For this review, take the finished solid that the model builds, in its own axes (mm). Face numbers are marked on the shaded views. A direction names the side the tool comes from. Coordinates: 2 decimals unless noted, no trailing zeros. Write each loop counter-clockwise with the first axis right and the second up, starting at its lowest first coordinate (ties: lowest second). Pieces come first, ordered by that corner, then holes. Notation, with made-up numbers: (4.25, -33.75) - (32.25, -33.75) arc R23 ccw to (32.25, -12.75) - close; hole circle Ø8 at (-18.75, 22.5). An arc over 180 degrees is marked (long way). Use one line per item in the form item = value. Start each with the question number.
1) We need section A-A (z = 31). Give the boundary of the cut face in (x, y), plus the area to 3 significant figures.
2) We need section D-D (x = 18.5). Give the boundary of the cut face in (y, z).
3) We need section C-C (y = -50). Give the boundary of the cut face in (x, z).
4) We need section B-B (x = 28.5). Give the boundary of the cut face in (y, z), plus the area to 3 significant figures.
5) For L1, parallel to X at y = -42, z = 25.5; L2, parallel to Z at x = 41.5, y = -10; L3, parallel to Y at x = 12, z = 3, list the stretches that pass through material, from the lowest coordinate up. Write a range as from..to.
6) Insertion check: P1, Ø3, axis at x = 32, y = -17, coming from the -Z side; P2, Ø19, axis at x = 39, z = 34, coming from the -Y side; P3, Ø5.5, axis at y = -21, z = 30.5, coming from the -X side; P4, Ø5, axis at x = 30.5, y = -36, coming from the +Z side. Each pin has a flat end and moves straight along its axis. Give the tip position at first contact, or say it passes through.
7) Tool access review of the marked faces 4, 5, 6 and 7: name each direction out of +Z, -Z, +X, -X, +Y, -Y from which nothing blocks a thin tool from reaching the whole face with its end or side.
8) Mouldability with a two-part tool opening along Y and no side actions: class the marked faces 1, 2 and 3 as pulls with the +Y half, pulls with the -Y half, needs draft (parallel to the pull), parting line crosses it, or undercut.
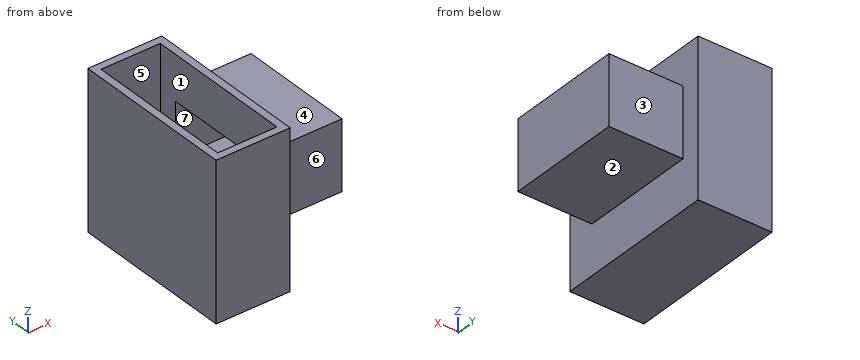
```python
from build123d import *

# Parameters (mm, degrees)
F0_W     = 35.9010435641
F0_H     = 59.8467253149
F1_DEPTH = 25.4
F2_W     = 56.2424324453
F2_H     = 53.3904395998
F3_DEPTH = 25.4
F4_W     = 39.9578805082
F4_H     = 23.749506101
F5_DEPTH = 25.4
F6_T     = -2.54


with BuildPart() as f1:
    # F0 (on Top) → F1 (new body)
    with BuildSketch(Plane.XY):
        with Locations((-17.950521782, 29.9233626574)):
            Rectangle(F0_W, F0_H)
    extrude(amount=F1_DEPTH)


with BuildPart() as f3:
    # F2 (on Right) → F3 (new body)
    with BuildSketch(Plane.YZ):
        with Locations((-28.1212162226, 26.6952197999)):
            Rectangle(F2_W, F2_H)
    extrude(amount=F3_DEPTH)

    # F4 (on face) → F5 (join)
    with BuildSketch(Plane.YZ.offset(25.4)):
        with Locations((-26.5757592861, 28.7435064092)):
            Rectangle(F4_W, F4_H)
    extrude(amount=F5_DEPTH)

    # F6
    f6_openings = [f3.faces().sort_by_distance(p)[0] for p in [
        (12.7, -28.121216, 53.39044),
    ]]
    offset(amount=F6_T, openings=f6_openings, kind=Kind.INTERSECTION)


solid = f3.part
```
Determined:
q1.outline = (0, -56.24) - (25.4, -56.24) - (25.4, -46.55) - (50.8, -46.55) - (50.8, -6.6) - (25.4, -6.6) - (25.4, 0) - (0, 0) - close; hole (2.54, -53.7) - (22.86, -53.7) - (22.86, -44.01) - (48.26, -44.01) - (48.26, -9.14) - (22.86, -9.14) - (22.86, -2.54) - (2.54, -2.54) - close
q1.area = 518 mm²
q2.outline = (-56.24, 0) - (0, 0) - (0, 53.39) - (-2.54, 53.39) - (-2.54, 2.54) - (-53.7, 2.54) - (-53.7, 53.39) - (-56.24, 53.39) - close
q3.outline = (0, 0) - (25.4, 0) - (25.4, 53.39) - (22.86, 53.39) - (22.86, 2.54) - (2.54, 2.54) - (2.54, 53.39) - (0, 53.39) - close
q4.outline = (-46.55, 16.87) - (-6.6, 16.87) - (-6.6, 40.62) - (-46.55, 40.62) - close; hole (-44.01, 19.41) - (-9.14, 19.41) - (-9.14, 38.08) - (-44.01, 38.08) - close
q4.area = 298 mm²
q5.L1 = 0..2.54, 48.26..50.8
q5.L2 = 16.87..19.41, 38.08..40.62
q5.L3 = -56.24..-53.7, -2.54..0
q6.P1 = 16.87
q6.P2 = -46.55
q6.P3 = 0
q6.P4 = 40.62
q7.face_4 = +Z, +X, +Y, -Y
q7.face_5 = +Z
q7.face_6 = +Z, -Z, +X, -Y
q7.face_7 = none
q8.face_1 = undercut
q8.face_2 = needs draft
q8.face_3 = pulls with the +Y half
